Build history of the part. All positions in model axes, mm. Give positions to 0.01 mm unless a question says otherwise; leave off trailing zeros. Loops run counter-clockwise (first coordinate to the right, second up) from the corner with the lowest first, then second, coordinate; pieces in that order, holes last. Notation, with made-up numbers: M 1,-24 L 46,-24 A20 cw 46,11 Z; hole C 16,28 d9. An arc over 180 degrees is marked long. Put each result on its own line as item: value.
```python
from build123d import *

# Parameters (mm, degrees)
CROQUIS1_W              = 75
CROQUIS1_H              = 24.5
CROQUIS1_R              = 2.5
SALIENTE_EXTRUIR1_DEPTH = 4


with BuildPart() as part:
    # Croquis1 → Saliente-Extruir1 (new body)
    with BuildSketch(Plane.XY):
        Rectangle(CROQUIS1_W, CROQUIS1_H)
        Circle(CROQUIS1_R, mode=Mode.SUBTRACT)
        with Locations((7, 4)):
            Circle(CROQUIS1_R, mode=Mode.SUBTRACT)
        with Locations(Location((7, -4, 0), (0, 0, 180))):
            Circle(CROQUIS1_R, mode=Mode.SUBTRACT)
        with Locations((-7, -4)):
            Circle(CROQUIS1_R, mode=Mode.SUBTRACT)
        with Locations(Location((-7, 4, 0), (0, 0, 180))):
            Circle(CROQUIS1_R, mode=Mode.SUBTRACT)
    extrude(amount=SALIENTE_EXTRUIR1_DEPTH)


solid = part.part
```
Q1. Slice it at B-B (y = 0). List the corners of the cut face in (x, z).
Here are the results:
outline: M -37.5,0 L -2.5,0 L -2.5,4 L -37.5,4 Z; M 2.5,0 L 37.5,0 L 37.5,4 L 2.5,4 Z
Q2. Slice it at D-D (z = 3.05). List the corners of the cut face in (x, y).
Here are the results:
outline: M -37.5,-12.25 L 37.5,-12.25 L 37.5,12.25 L -37.5,12.25 Z; hole C -7,-4 d5; hole C -7,4 d5; hole C 0,0 d5; hole C 7,-4 d5; hole C 7,4 d5
Q3. Probe line 1 (Y direction, x = -7, z = 2.25); line 2 (Y direction, x = 5, z = 1.1); line 3 (X direction, y = 5.25, z = 2.25). List the from-to ranges inside material, lowest first. Write a range as from..to.
Here are the results:
line 1: -12.25..-6.5, -1.5..1.5, 6.5..12.25
line 2: -12.25..-5.5, -2.5..2.5, 5.5..12.25
line 3: -37.5..-9.17, -4.83..4.83, 9.17..37.5
Q4. Mould opens along Y. For faces 1 (the flat face through (-1, 3, 0)), 2 (the cylindrical face through (4.615, -4.751, 1.972)), 3 (the cylindrical face through (-9.385, 3.249, 1.972)), 4 (the flat face through (-1, -12.25, 2)) say: pulls with the +Y half, pulls with the -Y half, needs draft (parallel to the pull), parting line crosses it, or undercut.
Here are the results:
face 1: needs draft
face 2: undercut
face 3: undercut
face 4: pulls with the -Y half
Q5. Slice it at C-C (y = -4). List the corners of the cut face in (x, z), and give its area (3 significant figures).
Here are the results:
outline: M -37.5,0 L -9.5,0 L -9.5,4 L -37.5,4 Z; M -4.5,0 L 4.5,0 L 4.5,4 L -4.5,4 Z; M 9.5,0 L 37.5,0 L 37.5,4 L 9.5,4 Z
area: 260 mm²
Q6. Slice it at A-A (x = 7). List the corners of the cut face in (y, z), and give its area (3 significant figures).
Here are the results:
outline: M -12.25,0 L -6.5,0 L -6.5,4 L -12.25,4 Z; M -1.5,0 L 1.5,0 L 1.5,4 L -1.5,4 Z; M 6.5,0 L 12.25,0 L 12.25,4 L 6.5,4 Z
area: 58.0 mm²
